Build history of the part. All positions in model axes, mm. Give positions to 0.01 mm unless a question says otherwise; leave off trailing zeros. Loops run counter-clockwise (first coordinate to the right, second up) from the corner with the lowest first, then second, coordinate; pieces in that order, holes last. Notation, with made-up numbers: (80, 68.25) -> (86, 68.25) arc R19 cw to (86, 86.25) -> close; hole circle Ø4 at (53.5, -2). An arc over 180 degrees is marked (long way). One line per question, with ' | ' between items. Start each with the question number.
(1) Slice it at B-B, the plane y = 14.5. Write the cut outline in (x, z).
(2) Drill centre lines: L1, parallel to X at y = 17.5, z = 0.55; L2, parallel to X at y = -3, z = 0.65; L3, parallel to Y at x = -23, z = 2.2. Where is each one in solid material? Low to high. Write a range as from..to.
(3) Slice it at D-D, the plane z = 1.8. Give the number of separate pieces and of enclosed holes in the cut face, then the cut area to 3 significant figures.
(4) Flat gauge pins, fed straight in: pin 1 Ø1 at (x, z) = (-21.5, 0.5) entering from +Y; pin 2 Ø1 at (y, z) = (16.5, 1) entering from -X; pin 3 Ø1.5 at (x, z) = (-2.5, 1) entering from +Y. Where does each tip first touch, or does it go through?
(5) Slice it at A-A, the plane x = -23. Write the cut outline in (y, z), then the cut area to 3 significant figures.
(6) Slice it at C-C, the plane x = -50. Write the cut outline in (y, z).
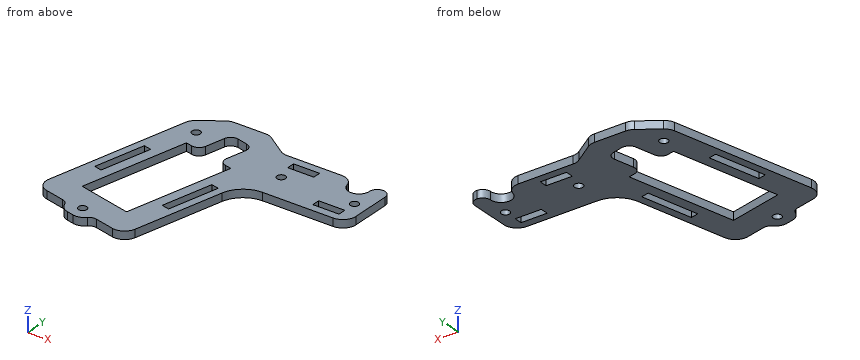
```python
from build123d import *

# Parameters (mm, degrees)
ESBO_O1_R                = 1.6000000000000096
ESBO_O1_R_2              = 1.5999999999999985
ESBO_O1_R_3              = 1.6000000000000019
ESBO_O1_R_4              = 1.6000000000000474
RESSALTO_EXTRUS_O1_DEPTH = 3
FILETE1_R                = 5
FILETE3_R                = 3
FILETE4_R                = 10
FILETE2_R                = 5


with BuildPart() as part:
    # Esboço1 → Ressalto-extrusão1 (new body)
    with BuildSketch(Plane.XY):
        with BuildLine():
            Line((-2.645751311064564, 23.000000000000014), (-31.296028057599443, 23.000000000000004))
            Line((-31.296028057599443, 22.999999999999996), (-41.49853289297047, 29.999999999999996))
            Line((-41.49853289297047, 29.999999999999996), (-56.49853289297047, 29.999999999999996))
            Line((-56.49853289297047, 29.999999999999996), (-66.7010377283415, 23.000000000000014))
            Line((-66.7010377283415, 23.000000000000014), (-80.74287914122172, -37.388961654722316))
            Line((-80.74287914122172, -37.388961654722316), (-65.64563872754113, -40.89942200794237))
            Line((-65.64563872754113, -40.89942200794238), (-66.49494365170727, -44.55198017254248))
            Line((-66.49494365170727, -44.55198017254248), (-56.754788546106894, -46.81679330365219))
            Line((-56.754788546106894, -46.81679330365219), (-55.90548362194077, -43.164235139052074))
            Line((-55.90548362194077, -43.164235139052074), (-40.80824320826024, -46.67469549227213))
            Line((-40.80824320826024, -46.67469549227213), (-29.955288394361567, 0))
            Line((-29.955288394361567, 0), (10, 0))
            Line((10.000000000000002, 0), (10.000000000000002, 23))
            Line((10.000000000000002, 23), (2.6457513110645188, 23.000000000000036))
            ThreePointArc((2.6457513110645325, 23.00000000000005), (2.416e-14, 16), (-2.645751311064569, 23.000000000000018))
        make_face()
        with Locations((-60.49245953335222, -40.81430918529715)):
            Circle(ESBO_O1_R, mode=Mode.SUBTRACT)
        Polygon((-34.44455590239048, -6.060615619977682), (-38.97418216460989, -25.54092583117841), (-41.89622869629002, -24.861481891845507), (-37.36660243407061, -5.381171680644762), align=None, mode=Mode.SUBTRACT)
        Polygon((-70.1426785025311, -18.293523811627356), (-73.06472503421121, -17.61407987229443), (-68.53509877199181, 1.8662303389063053), (-65.61305224031169, 1.1867863995733905), align=None, mode=Mode.SUBTRACT)
        Polygon((-53.86861044577067, 9.749384541179593), (-50.787533444320594, 22.999999999999996), (-41.04737833872022, 20.73518686889029), (-44.12845534017028, 7.484571410069881), (-38.771370032090054, 6.238924187959525), (-48.28358518275084, -34.669727255562044), (-68.73791090451164, -29.91361968023165), (-59.22569575385083, 10.995031763289926), align=None, mode=Mode.SUBTRACT)
        with Locations((-60.676910421506925, 17.999999999999996)):
            Circle(ESBO_O1_R_2, mode=Mode.SUBTRACT)
        Polygon((5.000000000000001, 6), (5, 3.0000000000000018), (-5, 2.9999999999999996), (-5.000000000000001, 5.999999999999999), align=None, mode=Mode.SUBTRACT)
        with Locations((-23.000000000000014, 10.999999999999996)):
            Circle(ESBO_O1_R_3, mode=Mode.SUBTRACT)
        Polygon((-14.999999999999993, 16.999999999999996), (-24.999999999999993, 16.999999999999993), (-24.999999999999993, 19.999999999999996), (-14.999999999999993, 19.999999999999996), align=None, mode=Mode.SUBTRACT)
        with Locations((5.000000000000001, 10.999999999999996)):
            Circle(ESBO_O1_R_4, mode=Mode.SUBTRACT)
    extrude(amount=RESSALTO_EXTRUS_O1_DEPTH)

    # Filete1
    filete1_edges = [part.edges().sort_by_distance(p)[0] for p in [
        (10, 0, 1.5),
        (-40.80824320826024, -46.67469549227213, 1.5),
        (-80.74287914122172, -37.388961654722316, 1.5),
    ]]
    fillet(filete1_edges, radius=FILETE1_R)

    # Filete3
    filete3_edges = [part.edges().sort_by_distance(p)[0] for p in [
        (-65.64563872754113, -40.89942200794238, 1.5),
        (-55.90548362194077, -43.164235139052074, 1.5),
        (2.6457513110645263, 23.000000000000043, 1.5),
        (10.000000000000002, 23, 1.5),
        (-50.787533444320594, 22.999999999999996, 1.5),
        (-41.04737833872022, 20.73518686889029, 1.5),
        (-44.12845534017028, 7.484571410069877, 1.5),
        (-53.86861044577067, 9.749384541179591, 1.5),
    ]]
    fillet(filete3_edges, radius=FILETE3_R - 0.0001)  # a hair under: the kernel refuses the full size

    # Filete4
    filete4_edges = [part.edges().sort_by_distance(p)[0] for p in [
        (-29.955288394361567, 0, 1.5),
    ]]
    fillet(filete4_edges, radius=FILETE4_R)

    # Filete2
    filete2_edges = [part.edges().sort_by_distance(p)[0] for p in [
        (-2.6457513110645667, 23.000000000000014, 1.5),
        (-56.754788546106894, -46.81679330365219, 1.5),
        (-66.49494365170727, -44.55198017254248, 1.5),
        (-31.296028057599443, 23, 1.5),
        (-41.49853289297047, 29.999999999999996, 1.5),
        (-56.49853289297047, 29.999999999999996, 1.5),
        (-66.7010377283415, 23.000000000000014, 1.5),
    ]]
    fillet(filete2_edges, radius=FILETE2_R - 0.0001)  # a hair under: the kernel refuses the full size


solid = part.part
```
Final values:
1) outline: (-68.68, 0) -> (-52.76, 0) -> (-52.76, 3) -> (-68.68, 3) -> close; (-42.5, 0) -> (10, 0) -> (10, 3) -> (-42.5, 3) -> close
2) L1: -67.98..-62.2, -59.16..-52.07, -41.8..-25, -15..-3.12, 3.12..10 | L2: -72.75..-69.67, -66.59..-62.48, -40.92..-29.16 | L3: -0.05..9.4, 12.6..17, 20..23
3) separate pieces: 1 | enclosed holes: 9 | area: 2,520 mm2
4) pin 1: y = 23 | pin 2: x = -68.33 | pin 3: y = 17.67
5) outline: (-0.05, 0) -> (9.4, 0) -> (9.4, 3) -> (-0.05, 3) -> close; (12.6, 0) -> (17, 0) -> (17, 3) -> (12.6, 3) -> close; (20, 0) -> (23, 0) -> (23, 3) -> (20, 3) -> close | area: 50.5 mm2
6) outline: (-44.54, 0) -> (-34.27, 0) -> (-34.27, 3) -> (-44.54, 3) -> close; (22.02, 0) -> (30, 0) -> (30, 3) -> (22.02, 3) -> close
